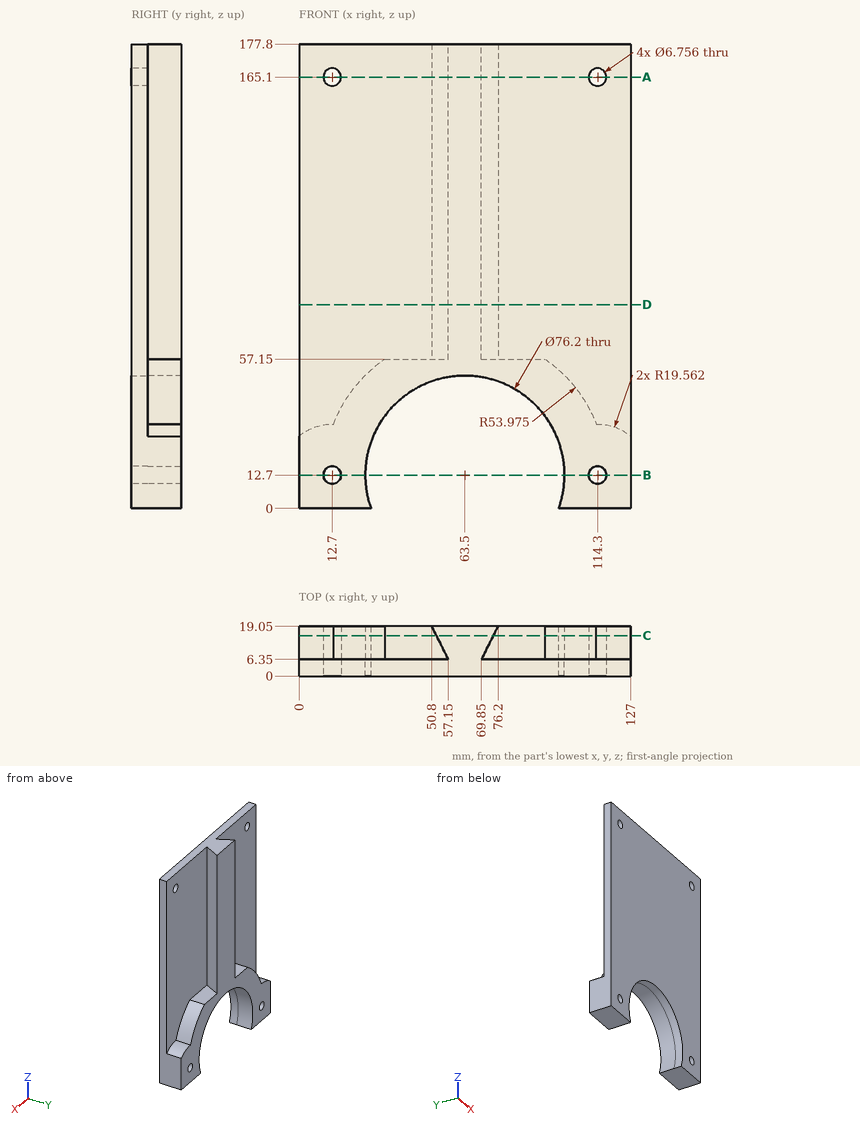
Verification items for this drawing (mm, ordinates from the low corner). Give positions to 0.01 mm unless a question says otherwise; leave off trailing zeros. Order: outer loops, then holes, each group sorted by start corner. A loop starts at its lowest first (then second) coordinate and runs counter-clockwise, first axis right, second up.
1) Cross-section at A-A (z = 165.1). Record the boundary of the cut face in (x, y).
Results are:
outline: (0, 0) - (9.32, 0) - (9.32, 6.35) - (0, 6.35) - close; (16.08, 0) - (110.92, 0) - (110.92, 6.35) - (69.85, 6.35) - (76.2, 19.05) - (50.8, 19.05) - (57.15, 6.35) - (16.08, 6.35) - close; (117.68, 0) - (127, 0) - (127, 6.35) - (117.68, 6.35) - close
2) Cross-section at C-C (y = 15.5). Give the number of separate pieces and of enclosed holes in the cut face, then the cut area to 3 significant figures.
Results are:
separate pieces: 1
enclosed holes: 2
area: 5,510 mm2
3) Gauge pin test, flat ends, axial feed: pin 1 (5 mm diameter, centred on x = 22, z = 140.5, fed in from +Y); pin 2 (10 mm diameter, centred on x = 42, y = 14.5, fed in from +Z). Record the tip position at first contact, or that the pin passes through.
Results are:
pin 1: stops at y = 6.35
pin 2: stops at z = 57.15
4) Cross-section at D-D (z = 78). Record the boundary of the cut face in (x, y), then the cut area to 3 significant figures.
Results are:
outline: (0, 0) - (127, 0) - (127, 6.35) - (69.85, 6.35) - (76.2, 19.05) - (50.8, 19.05) - (57.15, 6.35) - (0, 6.35) - close
area: 1,050 mm2
5) Cross-section at B-B (z = 12.7). Record the boundary of the cut face in (x, y).
Results are:
outline: (0, 0) - (9.32, 0) - (9.32, 19.05) - (0, 19.05) - close; (16.08, 0) - (25.4, 0) - (25.4, 19.05) - (16.08, 19.05) - close; (101.6, 0) - (110.92, 0) - (110.92, 19.05) - (101.6, 19.05) - close; (117.68, 0) - (127, 0) - (127, 19.05) - (117.68, 19.05) - close
6) Material ranges on probe 1 along Z at (x, y) = (12.7, 2.5); probe 2 along X at (y, z) = (9.75, 12.7); probe 3 along Z at (x, y) = (114.3, 16.25), recorded low to high.
Results are:
probe 1: z = 0 to 9.32, 16.08 to 161.72, 168.48 to 177.8
probe 2: x = 0 to 9.32, 16.08 to 25.4, 101.6 to 110.92, 117.68 to 127
probe 3: z = 0 to 9.32, 16.08 to 32.26
